The listing builds one solid part. Answer for the finished solid, in the listing's coordinates (mm). A direction names the side the tool comes from. Round coordinates to 2 decimals unless told otherwise and drop trailing zeros. Loops run counter-clockwise (first coordinate to the right, second up) from the corner with the lowest first, then second, coordinate; pieces in that order, holes last. Notation, with made-up numbers: (-11.75, -28) -> (-0.75, -28) arc R17 ccw to (-0.75, -18) -> close; hole circle Ø3 at (48, -1). An arc over 180 degrees is marked (long way). One line per question, with ' | ' between items.
from build123d import *

# Parameters (mm, degrees)
SKETCH1_W           = 85.8
SKETCH1_H           = 85.8
SKETCH1_R           = 3.3
BOSS_EXTRUDE1_DEPTH = 150
SKETCH2_R           = 34.8
BOSS_EXTRUDE2_DEPTH = 1.6
SKETCH3_R           = 7
BOSS_EXTRUDE3_DEPTH = 37
CUT_EXTRUDE1_START  = -10
CUT_EXTRUDE1_DEPTH  = 157
FILLET1_R           = 5
FILLET2_R           = 3


with BuildPart() as part:
    # Sketch1 → Boss-Extrude1 (new body)
    with BuildSketch(Plane(origin=(0, 0, 0), x_dir=(1, 0, 0), z_dir=(0, 1, 0))):
        Rectangle(SKETCH1_W, SKETCH1_H)
        with Locations(Location((-34.8, 34.8, 0), (0, 0, 270))):
            Circle(SKETCH1_R, mode=Mode.SUBTRACT)
        with Locations(Location((34.8, 34.8, 0), (0, 0, 270))):
            Circle(SKETCH1_R, mode=Mode.SUBTRACT)
        with Locations(Location((34.8, -34.8, 0), (0, 0, 270))):
            Circle(SKETCH1_R, mode=Mode.SUBTRACT)
        with Locations(Location((-34.8, -34.8, 0), (0, 0, 270))):
            Circle(SKETCH1_R, mode=Mode.SUBTRACT)
    extrude(amount=-BOSS_EXTRUDE1_DEPTH)

    # Sketch2 → Boss-Extrude2 (add)
    with BuildSketch(Plane(origin=(0, 0, 0), x_dir=(1, 0, 0), z_dir=(0, 1, 0))):
        with Locations(Location((0, 0, 0), (0, 0, 90))):
            Circle(SKETCH2_R)
    extrude(amount=BOSS_EXTRUDE2_DEPTH)

    # Sketch3 → Boss-Extrude3 (add)
    with BuildSketch(Plane(origin=(0, 0, 0), x_dir=(1, 0, 0), z_dir=(0, 1, 0))):
        with Locations(Location((0, 0, 0), (0, 0, 270))):
            Circle(SKETCH3_R)
    extrude(amount=BOSS_EXTRUDE3_DEPTH)

    # Sketch4 → Cut-Extrude1 (cut)
    with BuildSketch(Plane(origin=(0, 0, 0), x_dir=(1, 0, 0), z_dir=(0, 1, 0)).offset(CUT_EXTRUDE1_START)):
        with BuildLine():
            Line((-34.8, 28.8), (-51.295140444, 28.8))
            Line((-51.295140444, 28.8), (-51.295140444, 48.66224904))
            Line((-51.295140444, 48.66224904), (-28.8, 48.66224904))
            Line((-28.8, 48.66224904), (-28.8, 34.8))
            ThreePointArc((-28.8, 34.8), (-30.557359313, 30.557359313), (-34.8, 28.8))
        make_face()
        with BuildLine():
            Line((48.66224904, 28.8), (34.8, 28.8))
            ThreePointArc((34.8, 28.8), (30.557359313, 30.557359313), (28.8, 34.8))
            Line((28.8, 34.8), (28.8, 51.295140444))
            Line((28.8, 51.295140444), (48.66224904, 51.295140444))
            Line((48.66224904, 51.295140444), (48.66224904, 28.8))
        make_face()
        with BuildLine():
            Line((28.8, -48.66224904), (28.8, -34.8))
            ThreePointArc((28.8, -34.8), (30.557359313, -30.557359313), (34.8, -28.8))
            Line((34.8, -28.8), (51.295140444, -28.8))
            Line((51.295140444, -28.8), (51.295140444, -48.66224904))
            Line((51.295140444, -48.66224904), (28.8, -48.66224904))
        make_face()
        with BuildLine():
            Line((-48.66224904, -28.8), (-34.8, -28.8))
            ThreePointArc((-34.8, -28.8), (-30.557359313, -30.557359313), (-28.8, -34.8))
            Line((-28.8, -34.8), (-28.8, -51.295140444))
            Line((-28.8, -51.295140444), (-48.66224904, -51.295140444))
            Line((-48.66224904, -51.295140444), (-48.66224904, -28.8))
        make_face()
    extrude(amount=-CUT_EXTRUDE1_DEPTH, mode=Mode.SUBTRACT)

    # Fillet1
    fillet1_edges = [part.edges().sort_by_distance(p)[0] for p in [
        (42.9, -5, -42.9),
        (-42.9, -5, -42.9),
        (-42.9, -5, 42.9),
        (42.9, -5, 42.9),
    ]]
    fillet(fillet1_edges, radius=FILLET1_R)

    # Fillet2
    fillet2_edges = [part.edges().sort_by_distance(p)[0] for p in [
        (-28.8, -80, 42.9),
        (-42.9, -80, 28.8),
        (42.9, -80, 28.8),
        (28.8, -80, 42.9),
        (28.8, -80, -42.9),
        (42.9, -80, -28.8),
        (-42.9, -80, -28.8),
        (-28.8, -80, -42.9),
    ]]
    fillet(fillet2_edges, radius=FILLET2_R)


solid = part.part
Q1. A cutting plane is placed at D-D on z = -13.5. Give the vertices of the cut face in (x, y).
Numbers:
outline: (-42.9, -150) -> (42.9, -150) -> (42.9, 0) -> (32.07, 0) -> (32.07, 1.6) -> (-32.07, 1.6) -> (-32.07, 0) -> (-42.9, 0) -> close
Q2. For faces 1 (the face through (-37, -79, 28.8)), 2 (the face through (-36.1, -10, -38.3)), 3 (the face through (30.511, -79.02, 30.604)), determine the directions among +Z, -Z, +X, -X, +Y, -Y from which every point of the face is accessible in a straight line to the end or side of a thin tool.
Numbers:
face 1: +Z, -X, -Y | face 2: -Z, -X, -Y | face 3: +Z, +X, -Y
Q3. Find the intervals of material crossed by line 1 (X direction, y = -7.5, z = 34.8); line 2 (Z direction, x = -34, y = -3), in increasing order. Write a range as from..to.
Numbers:
line 1: -42.9..-38.1, -31.5..31.5, 38.1..42.9 | line 2: -42.9..-38, -31.6..31.6, 38..42.9
Q4. Given pin 1 Ø5.5 at (y, z) = (-52, 36.5) entering from -X; pin 2 Ø5.5 at (x, y) = (-37.5, -59) entering from +Z; pin 3 Ø5 at (x, z) = (27, -13) entering from +Y; pin 4 Ø13.5 at (x, z) = (31, -30.5) entering from -Y, each flat-ended and moving along its own axis, determine where each tip first touches the part or whether it passes through.
Numbers:
pin 1: x = -28.89 | pin 2: z = 28.8 | pin 3: y = 1.6 | pin 4: y = -150
Q5. A cutting plane is placed at B-B on z = 0. Give the vertices of the cut face in (x, y), plus the area to 3 significant figures.
Numbers:
outline: (-42.9, -150) -> (42.9, -150) -> (42.9, 0) -> (34.8, 0) -> (34.8, 1.6) -> (7, 1.6) -> (7, 37) -> (-7, 37) -> (-7, 1.6) -> (-34.8, 1.6) -> (-34.8, 0) -> (-42.9, 0) -> close | area: 13,500 mm^2
Q6. For a pull along Z with two mould halves and no side action, classify faces 4 (the face through (-28.8, -79, -37)), 5 (the face through (30.604, -79.02, -30.511)), 6 (the face through (-36.808, -4.93, -37.419)) as pulls with the +Z half, pulls with the -Z half, needs draft (parallel to the pull), parting line crosses it, or undercut.
Numbers:
face 4: needs draft | face 5: pulls with the -Z half | face 6: undercut
Q7. A cutting plane is placed at C-C on y = -91. Give the vertices of the cut face in (x, z).
Numbers:
outline: (-42.9, -25.8) arc R3 ccw to (-39.9, -28.8) -> (-34.8, -28.8) arc R6 cw to (-28.8, -34.8) -> (-28.8, -39.9) arc R3 ccw to (-25.8, -42.9) -> (25.8, -42.9) arc R3 ccw to (28.8, -39.9) -> (28.8, -34.8) arc R6 cw to (34.8, -28.8) -> (39.9, -28.8) arc R3 ccw to (42.9, -25.8) -> (42.9, 25.8) arc R3 ccw to (39.9, 28.8) -> (34.8, 28.8) arc R6 cw to (28.8, 34.8) -> (28.8, 39.9) arc R3 ccw to (25.8, 42.9) -> (-25.8, 42.9) arc R3 ccw to (-28.8, 39.9) -> (-28.8, 34.8) arc R6 cw to (-34.8, 28.8) -> (-39.9, 28.8) arc R3 ccw to (-42.9, 25.8) -> close
Q8. A cutting plane is placed at A-A on x = 0. Give the vertices of the cut face in (y, z).
Numbers:
outline: (-150, -42.9) -> (0, -42.9) -> (0, -34.8) -> (1.6, -34.8) -> (1.6, -7) -> (37, -7) -> (37, 7) -> (1.6, 7) -> (1.6, 34.8) -> (0, 34.8) -> (0, 42.9) -> (-150, 42.9) -> close
